from build123d import *

# Parameters (mm, degrees)
SKETCH3_W               = 37.4904
SKETCH3_H               = 74.9808
SKETCH3_W_2             = 7.8613
SKETCH3_H_2             = 37.4904
CUT_EXTRUDE1_DEPTH      = 12.7
HOLE1_D                 = 4.7625
HOLE1_DEPTH             = 17.4625
HOLE1_TIP               = 1.374815329
SKETCH8_R               = 2.0193
CUT_EXTRUDE2_DEPTH      = 5.895975
CUT_EXTRUDE2_DEPTH_BACK = 5.895975


with BuildPart() as part:
    # Sketch1 → Revolve1 (revolve)
    with BuildSketch(Plane.XY):
        Polygon((0, 0), (0, 4.90855), (0.762, 5.67055), (3.7592, 5.67055), (4.2672, 5.16255), (4.7752, 5.16255), (4.7752, 6.16585), (7.9502, 6.16585), (7.9502, 8.6106), (8.7122, 9.3726), (16.7132, 9.3726), (17.4752, 8.6106), (17.4752, 0), align=None)
    revolve(axis=Axis((17.4752, 0, 0), (-1, 0, 0)))

    # Sketch2 → Revolve2 (revolve)
    with BuildSketch(Plane.XY):
        with BuildLine():
            Line((17.4752, 0), (17.4752, 5.5245))
            Line((17.4752, 5.5245), (18.7452, 5.5245))
            Line((18.7452, 5.5245), (18.7452, 5.3721))
            ThreePointArc((18.7452, 5.3721), (18.979543864, 4.806343864), (19.5453, 4.572))
            Line((19.5453, 4.572), (20.7137, 4.572))
            ThreePointArc((20.7137, 4.572), (20.9804, 4.617758486), (21.216594343, 4.7498))
            Line((21.216594343, 4.7498), (21.279456136, 4.8006))
            Line((21.279456136, 4.8006), (22.035106136, 5.55625))
            Line((22.035106136, 5.55625), (29.41955, 5.55625))
            Line((29.41955, 5.55625), (30.1752, 4.8006))
            Line((30.1752, 4.8006), (30.1752, 0))
            Line((30.1752, 0), (17.4752, 0))
        make_face()
    revolve(axis=Axis((30.1752, 0, 0), (-1, 0, 0)))

    # Sketch3 → Cut-Extrude1 (cut)
    with BuildSketch(Plane(origin=(30.1752, 0, 0), x_dir=(0, 0, -1), z_dir=(1, 0, 0))):
        Rectangle(SKETCH3_W, SKETCH3_H)
        Rectangle(SKETCH3_W_2, SKETCH3_H_2, mode=Mode.SUBTRACT)
    extrude(amount=-CUT_EXTRUDE1_DEPTH, mode=Mode.SUBTRACT)

    # Hole1
    with Locations(Plane.ZY):
        with Locations((0, 0)):
            Hole(HOLE1_D / 2, depth=HOLE1_DEPTH)
            with Locations((0, 0, -(HOLE1_DEPTH + HOLE1_TIP / 2))):  # 120° drill point
                Cone(0, HOLE1_D / 2, HOLE1_TIP, mode=Mode.SUBTRACT)

    # Sketch6 → Cut-Revolve1 (revolve, cut)
    with BuildSketch(Plane(origin=(0, 0, 0), x_dir=(1, 0, 0), z_dir=(0, 1, 0))):
        Polygon((12.7, 0), (14.68374, 0), (14.68374, -7.92734), (15.113, -8.3566), (16.6624, -8.3566), (16.6624, -9.3726), (12.7, -9.3726), align=None)
    revolve(axis=Axis((12.7, 0, 9.3726), (0, 0, -1)), mode=Mode.SUBTRACT)

    # Sketch7 → Revolve3 (revolve)
    with BuildSketch(Plane.XY):
        with BuildLine():
            Line((4.066488686, 6.081681804), (4.663607684, 5.484562806))
            ThreePointArc((4.663607684, 5.484562806), (4.700805122, 5.394760245), (4.663607684, 5.304957684))
            Line((4.663607684, 5.304957684), (4.5212, 5.16255))
            Line((4.5212, 5.16255), (4.2672, 5.16255))
            Line((4.2672, 5.16255), (4.2672, 4.90855))
            Line((4.2672, 4.90855), (4.7752, 4.90855))
            Line((4.7752, 4.90855), (4.7752, 5.660338686))
            Line((4.7752, 5.660338686), (4.269688686, 6.16585))
            Line((4.269688686, 6.16585), (4.066488686, 6.16585))
            Line((4.066488686, 6.16585), (4.066488686, 6.081681804))
        make_face()
    revolve(axis=Axis((4.7752, 0, 0), (-1, 0, 0)))

    # Sketch8 → Cut-Extrude2 (cut, two sides)
    with BuildSketch(Plane.XY) as cut_extrude2_sk:
        with Locations((23.8252, 0)):
            Circle(SKETCH8_R)
    extrude(amount=CUT_EXTRUDE2_DEPTH, mode=Mode.SUBTRACT)
    extrude(cut_extrude2_sk.sketch, amount=-CUT_EXTRUDE2_DEPTH_BACK, mode=Mode.SUBTRACT)


solid = part.part
Verification items for the finished model (mm, model axes). A direction names the side the tool comes from. Coordinates: 2 decimals unless noted, no trailing zeros. Write each loop counter-clockwise with the first axis right and the second up, starting at its lowest first coordinate (ties: lowest second). Pieces come first, ordered by that corner, then holes. Notation, with made-up numbers: (65.25, 77) - (86.25, 77) arc R15 cw to (86.25, 84) - close; hole circle Ø4 at (60.5, 87.25). An arc over 180 degrees is marked (long way). Answer as a JSON object with one key per item and string values.
(1) Cross-section at A-A on x = 25.5. Record the cut outline in (y, z), plus the area to 3 significant figures.
Report:
{"outline": "(-3.93, -3.93) - (-1.13, -3.93) - (-1.13, 3.93) - (-3.93, 3.93) arc R5.56 ccw to start; (1.13, -3.93) - (3.93, -3.93) arc R5.56 ccw to (3.93, 3.93) - (1.13, 3.93) - close", "area": "61.7 mm^2"}
(2) Cross-section at C-C on z = 2.75. Give the number of separate pieces and of enclosed holes in the cut face, plus the area to 3 significant figures.
Report:
{"separate pieces": "1", "enclosed holes": "2", "area": "341 mm^2"}
(3) Thickness scan on line 1 along X through (y, z) = (1.75, 2); line 2 along Y through (x, z) = (12, 0); line 3 along Z through (x, y) = (28.5, -3.25). Record the ranges inside material, lowest first.
Report:
{"line 1": "0 to 11.77, 13.63 to 22.82, 24.83 to 30.18", "line 2": "-9.37 to -2.38, 2.38 to 9.37", "line 3": "-3.93 to 3.93"}
(4) Gauge pin test, flat ends, axial feed: pin 1 Ø6.5 at (x, y) = (12.7, 0) entering from +Z; pin 2 Ø2 at (y, z) = (-5, 0.5) entering from +X; pin 3 Ø6 at (x, z) = (24.5, -2.5) entering from +Y; pin 4 Ø6 at (x, y) = (19.5, 4.5) entering from -Z. Record the tip position at first contact, or that the pin passes through.
Report:
{"pin 1": "z = 8.36", "pin 2": "x = 30.18", "pin 3": "y = 5.56", "pin 4": "z = -8.74"}
(5) Tool access check on faces 1 (the conical face through (21.41, -4.93, -0.07)), 2 (the conical face through (30.055, 4.921, 0.066)), 3 (the flat face through (25, 2, 3.931)), 4 (the cylindrical face through (2.282, -0.738, -5.622)), 5 (the cylindrical face through (9.556, 2.411, 8.759)). Record the directions out of +Z, -Z, +X, -X, +Y, -Y that give a thin tool (end or side, any length) a straight path to the whole face; none if there is none.
Report:
{"face 1": "-Y", "face 2": "+X, +Y", "face 3": "+Z, +X, +Y, -Y", "face 4": "-X", "face 5": "+Z"}
(6) Cross-section at B-B on x = 12.7. Record the cut outline in (y, z).
Report:
{"outline": "(-3.96, 8.36) - (-3.96, 8.49) arc R9.37 ccw (long way) to (3.96, 8.49) - (3.96, 8.36) - (2.41, 8.36) - (1.98, 7.93) - (1.98, 1.32) arc R2.38 cw (long way) to (-1.98, 1.32) - (-1.98, 7.93) - (-2.41, 8.36) - close"}
